Part model, mm, in its own coordinate system. Face numbers are marked on the shaded views. A direction names the side the tool comes from. Round coordinates to 2 decimals unless told otherwise and drop trailing zeros. Write each loop counter-clockwise with the first axis right and the second up, starting at its lowest first coordinate (ties: lowest second). Pieces come first, ordered by that corner, then holes. Notation, with made-up numbers: M 7,1 L 23,1 A15 ccw 23,25 Z; hole C -11,80 d9. An arc over 180 degrees is marked long. Answer as a JSON object with one key per item and string values. Group by question number.
1. Band-saw the part on D-D, the plane x = 9. Write the cut outline in (y, z) (3 decimals).
2. Band-saw the part on B-B, the plane z = -5. Write the cut outline in (x, y).
3. Drill centre lines: line 1 (Y direction, x = 7.5, z = -5); line 2 (Z direction, x = 9.65, y = 3.4); line 3 (Z direction, x = 5.25, y = 1) (3 decimals). Where is each one in solid material? Low to high. Write a range as from..to.
4. Two-plate mould, pull along Y, no slides. Class the marked faces 1, 2 and 3: +Y half, -Y half, draft (parallel to the pull), parting line (faces both ways), or undercut.
5. Band-saw the part on A-A, the plane x = 2.75. Write the cut outline in (y, z) (3 decimals), plus the area to 3 significant figures.
6. Band-saw the part on C-C, the plane x = 4.25. Write the cut outline in (y, z) (3 decimals).
7. Which spindle directions (+Z, -Z, +X, -X, +Y, -Y) get a long thin tool onto all of the face, cutting with end or side? Do the marked faces 4, 5, 6, 7 and 8. Say none if no direction does.
8. Drop flat-ended pins along their axis: pin 1 (1.5 mm diameter, centred on x = 3.5, z = -2.5, fed in from +Y); pin 2 (4.5 mm diameter, centred on y = 12, z = -3.5, fed in from -X); pin 3 (4 mm diameter, centred on x = 7, z = -3.5, fed in from -Y); pin 4 (4 mm diameter, centred on y = 5.5, z = -3.5, fed in from -X). Give the stop position or say it passes through.
from build123d import *

# Parameters (mm, degrees)
SKETCH1_W           = 10.16
SKETCH1_H           = 7.62
BOSS_EXTRUDE1_DEPTH = 13.97
SKETCH2_R           = 2.9
CUT_EXTRUDE1_DEPTH  = 1
CUT_EXTRUDE2_REACH  = 20.88
SKETCH3_W           = 4.81
SKETCH3_H           = 2
SKETCH5_W           = 4.81
SKETCH5_H           = 4.22
CUT_EXTRUDE4_DEPTH  = 5.5372
SKETCH6_W           = 4.81
SKETCH6_H           = 10.57
CUT_EXTRUDE6_DEPTH  = 2.9972
SKETCH7_W           = 4.81
SKETCH7_H           = 3.4
CUT_EXTRUDE7_DEPTH  = 5.5372


with BuildPart() as part:
    # Sketch1 → Boss-Extrude1 (new body)
    with BuildSketch(Plane(origin=(0, 0, 0), x_dir=(1, 0, 0), z_dir=(0, 1, 0))):
        with Locations((5.08, 3.81)):
            Rectangle(SKETCH1_W, SKETCH1_H)
    extrude(amount=BOSS_EXTRUDE1_DEPTH)

    # Sketch2 → Cut-Extrude1 (cut)
    with BuildSketch(Plane(origin=(10.16, 0, 0), x_dir=(0, 0, -1), z_dir=(1, 0, 0))):
        with Locations((4.008616611, 3.4)):
            Circle(SKETCH2_R)
        with Locations((3.81, 9.75)):
            Circle(SKETCH2_R)
    extrude(amount=-CUT_EXTRUDE1_DEPTH, mode=Mode.SUBTRACT)

    # Sketch3 → Cut-Extrude2 (cut, up to next)
    with BuildSketch(Plane(origin=(10.16, 0, 0), x_dir=(0, 0, -1), z_dir=(1, 0, 0)), mode=Mode.PRIVATE) as cut_extrude2_sk1:
        with BuildLine():
            Line((1.905, 3.9), (5.715, 3.9))
            ThreePointArc((5.715, 3.9), (6.215, 3.4), (5.715, 2.9))
            Line((5.715, 2.9), (1.905, 2.9))
            ThreePointArc((1.905, 2.9), (1.405, 3.4), (1.905, 3.9))
        make_face()
    cut_extrude2_tool1 = extrude(cut_extrude2_sk1.sketch, amount=-CUT_EXTRUDE2_REACH, mode=Mode.PRIVATE) & part.part
    # Sketch3 → Cut-Extrude2 (cut, up to next)
    with BuildSketch(Plane(origin=(10.16, 0, 0), x_dir=(0, 0, -1), z_dir=(1, 0, 0)), mode=Mode.PRIVATE) as cut_extrude2_sk2:
        with BuildLine():
            Line((1.905, 10.25), (5.715, 10.25))
            ThreePointArc((5.715, 10.25), (6.215, 9.75), (5.715, 9.25))
            Line((5.715, 9.25), (1.905, 9.25))
            ThreePointArc((1.905, 9.25), (1.405, 9.75), (1.905, 10.25))
        make_face()
    cut_extrude2_tool2 = extrude(cut_extrude2_sk2.sketch, amount=-CUT_EXTRUDE2_REACH, mode=Mode.PRIVATE) & part.part
    # Sketch3 → Cut-Extrude2 (cut, up to next)
    with BuildSketch(Plane(origin=(10.16, 0, 0), x_dir=(0, 0, -1), z_dir=(1, 0, 0)), mode=Mode.PRIVATE) as cut_extrude2_sk3:
        with Locations((3.81, 1)):
            Rectangle(SKETCH3_W, SKETCH3_H)
    cut_extrude2_tool3 = extrude(cut_extrude2_sk3.sketch, amount=-CUT_EXTRUDE2_REACH, mode=Mode.PRIVATE) & part.part
    add(cut_extrude2_tool1.solids().sort_by_distance((10.16, 3.4, -3.81))[0], mode=Mode.SUBTRACT)
    add(cut_extrude2_tool2.solids().sort_by_distance((10.16, 9.75, -3.81))[0], mode=Mode.SUBTRACT)
    add(cut_extrude2_tool3.solids().sort_by_distance((10.16, 1, -3.81))[0], mode=Mode.SUBTRACT)

    # Sketch5 → Cut-Extrude4 (cut)
    with BuildSketch(Plane.ZY):
        with Locations((-3.81, 11.86)):
            Rectangle(SKETCH5_W, SKETCH5_H)
    extrude(amount=-CUT_EXTRUDE4_DEPTH, mode=Mode.SUBTRACT)

    # Sketch6 → Cut-Extrude6 (cut)
    with BuildSketch(Plane.ZY):
        with Locations((-3.81, 8.685)):
            Rectangle(SKETCH6_W, SKETCH6_H)
    extrude(amount=-CUT_EXTRUDE6_DEPTH, mode=Mode.SUBTRACT)

    # Sketch7 → Cut-Extrude7 (cut)
    with BuildSketch(Plane.ZY):
        with Locations((-3.81, 1.7)):
            Rectangle(SKETCH7_W, SKETCH7_H)
    extrude(amount=-CUT_EXTRUDE7_DEPTH, mode=Mode.SUBTRACT)


solid = part.part
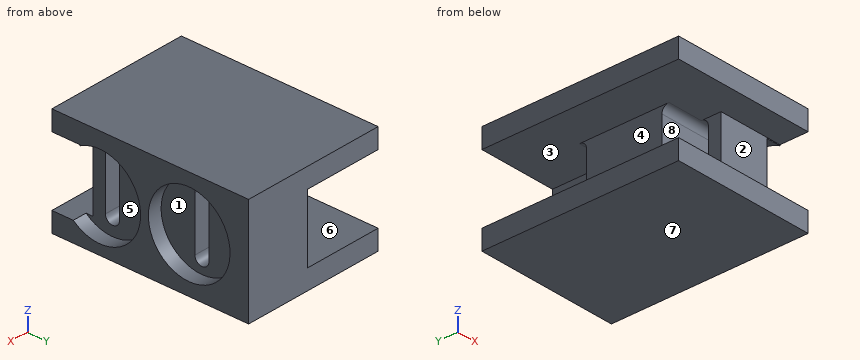
Worked answers:
{
 "1": {"outline": "M 0,-7.62 L 13.97,-7.62 L 13.97,0 L 0,0 L 0,-1.405 L 2,-1.405 L 2,-6.215 L 0,-6.215 Z; hole M 2.9,-5.715 A0.5 ccw 3.9,-5.715 L 3.9,-1.905 A0.5 ccw 2.9,-1.905 Z; hole M 9.25,-5.715 A0.5 ccw 10.25,-5.715 L 10.25,-1.905 A0.5 ccw 9.25,-1.905 Z"},
 "2": {"outline": "M 3,3.9 L 9.16,3.9 L 9.16,6.13 L 10.16,6.13 L 10.16,7.11 L 9.16,7.11 L 9.16,9.25 L 3,9.25 Z; M 5.54,2 L 9.16,2 L 9.16,2.9 L 5.54,2.9 Z; M 5.54,10.25 L 9.16,10.25 L 9.16,12.39 L 10.16,12.39 L 10.16,13.97 L 5.54,13.97 Z"},
 "3": {"line 1": "y = 2..2.9, 3.9..9.25, 10.25..13.97", "line 2": "z = -7.62..-6.91, -1.11..0", "line 3": "z = -7.62..-6.215, -1.405..0"},
 "4": {"face 1": "undercut", "face 2": "-Y half", "face 3": "draft"},
 "5": {"outline": "M 0,-7.62 L 13.97,-7.62 L 13.97,-6.215 L 0,-6.215 Z; M 0,-1.405 L 13.97,-1.405 L 13.97,0 L 0,0 Z", "area": "39.3 mm^2"},
 "6": {"outline": "M 0,-7.62 L 13.97,-7.62 L 13.97,-6.215 L 9.75,-6.215 A0.5 cw 9.25,-5.715 L 9.25,-1.905 A0.5 cw 9.75,-1.405 L 13.97,-1.405 L 13.97,0 L 0,0 L 0,-1.405 L 3.4,-1.405 A0.5 cw 3.9,-1.905 L 3.9,-5.715 A0.5 cw 3.4,-6.215 L 0,-6.215 Z"},
 "7": {"face 4": "-X, +Y, -Y", "face 5": "+X", "face 6": "-X", "face 7": "-Z, +X, -X, +Y, -Y", "face 8": "+X, -X"},
 "8": {"pin 1": "stops at y = 9.27", "pin 2": "stops at x = 0", "pin 3": "stops at y = 2", "pin 4": "stops at x = 3"}
}
